```python
from build123d import *


# Read off the part's stored shape, not the designer's step: Shell1
with BuildPart() as part:
    # Sketch1 → Revolve1 (revolve)
    with BuildSketch(Plane(origin=(0, 0, 0), x_dir=(0, 0, -1), z_dir=(1, 0, 0)), mode=Mode.PRIVATE) as revolve1_sk:
        with BuildLine():
            Line((0.74336912, 4.5), (12.74336912, 4.5))
            ThreePointArc((12.74336912, 4.5), (18.035165187, 8.916407865), (24.74336912, 10.5))
            Line((24.74336912, 10.5), (80.74336912, 10.5))
            ThreePointArc((80.74336912, 10.5), (88.167990322, 7.424621202), (91.24336912, 0))
            Line((91.24336912, 0), (0.74336912, 0))
            Line((0.74336912, 0), (0.74336912, 4.5))
        make_face()
    revolve(revolve1_sk.sketch.rotate(Axis((0, 0, 0), (0, 0, -1)), 90), axis=Axis((0, 0, 0), (0, 0, -1)))

    # Shell1 outline → Shell1 (revolve, cut)
    with BuildSketch(Plane.XZ):
        with BuildLine():
            Line((0, -0.74336912), (0, -90.24336912))
            ThreePointArc((0, -90.24336912), (6.717514422, -87.46088354), (9.5, -80.743369117))
            Line((9.5, -80.743369117), (9.5, -24.74336912))
            ThreePointArc((9.5, -24.74336912), (7.909673646, -18.262628421), (3.5, -13.254243826))
            Line((3.5, -13.254243826), (3.5, -0.74336912))
            Line((3.5, -0.74336912), (0, -0.74336912))
        make_face()
    revolve(axis=Axis((0, 0, 0), (0, 0, 1)), mode=Mode.SUBTRACT)


solid = part.part
```
CAD build for the part. Positions are in the model's coordinates, mm. A direction names the side the tool comes from. Coordinates: 2 decimals unless noted, no trailing zeros. Order: outer loops, then holes, each group sorted by start corner. A loop starts at its lowest first (then second) coordinate and runs counter-clockwise, first axis right, second up. Notation, with made-up numbers: (78, 7.5) -> (114, 7.5) arc R22 ccw to (114, 43.5) -> close; hole circle Ø5 at (69.25, 20). An arc over 180 degrees is marked (long way). Use one line per item in the form item = value. Start each with the question number.
1) Drop flat-ended pins along their axis: pin 1 (1.5 mm diameter, centred on y = 2.5, z = -36.5, fed in from -X); pin 2 (1.5 mm diameter, centred on x = 1, z = -33.5, fed in from -Y); pin 3 (5 mm diameter, centred on x = 2.5, y = 4, fed in from -Z); pin 4 (4 mm diameter, centred on y = 0.5, z = -32, fed in from -X). Give the stop position or say it passes through.
2) Drill centre lines: L1, parallel to X at y = 0.5, z = -73; L2, parallel to Y at x = 0, z = -7; L3, parallel to Z at x = -8.25, y = -0.5. Where is each one in solid material? Low to high. Write a range as [from, to].
3) Pull direction X, two halves, no side cores. Call faces 1 (the cylindrical face through (-3.32, -3.04, -6.83)), 2 (the cylindrical face through (4.38, -8.43, -52.35)), 3 (the flat face through (0, 4, -0.743)): +X half, -X half, draft (parallel to the pull), parting line (faces both ways), or undercut.
4) Band-saw the part on A-A on z = -6.5. Give the cut face in (x, y), then the cut area to 3 significant figures.
5) Tool access for faces 4 (the cylindrical face through (3.233, -1.341, -6.911)), 5 (the cylindrical face through (10, -3.2, -53.1)): list every direction of +Z, -Z, +X, -X, +Y, -Y with a clear straight run to the whole face (end or side of a thin tool).
6) Band-saw the part on B-B on z = -82.5. Give the cut face in (x, y), then the cut area to 3 significant figures.
Entries:
q1.pin_1 = -10.35
q1.pin_2 = -10.5
q1.pin_3 = -91.01
q1.pin_4 = -10.5
q2.L1 = [-10.49, -9.49], [9.49, 10.49]
q2.L2 = [-4.5, -3.5], [3.5, 4.5]
q2.L3 = [-87.22, -85.43], [-18.99, -16.87]
q3.face_1 = parting line
q3.face_2 = undercut
q3.face_3 = draft
q4.outline = circle Ø9 at (0, 0); hole circle Ø7 at (0, 0)
q4.area = 25.1 mm2
q5.face_4 = +Z
q5.face_5 = +Z, -Z
q6.outline = circle Ø20.7 at (0, 0); hole circle Ø18.67 at (0, 0)
q6.area = 62.8 mm2
